```python
from build123d import *

# Parameters (mm, degrees)
SKETCH1_W            = 31.75
SKETCH1_H            = 50.8
BOSS_EXTRUDE1_DEPTH  = 3.175
CUT_EXTRUDE1_REACH   = 32.121
SKETCH2_R            = 12.7
M4_CLEARANCE_HOLE1_D = 4.4958


with BuildPart() as part:
    # Sketch1 → Boss-Extrude1 (new body)
    with BuildSketch(Plane(origin=(0, 0, 0), x_dir=(1, 0, 0), z_dir=(0, 1, 0))):
        Rectangle(SKETCH1_W, SKETCH1_H)
    extrude(amount=BOSS_EXTRUDE1_DEPTH)

    # Sketch2 → Cut-Extrude1 (cut, up to next)
    with BuildSketch(Plane(origin=(0, 3.175, 0), x_dir=(1, 0, 0), z_dir=(0, 1, 0)), mode=Mode.PRIVATE) as cut_extrude1_sk1:
        with Locations(Location((0, 0, 0), (0, 0, 270))):
            Circle(SKETCH2_R)
    cut_extrude1_tool1 = extrude(cut_extrude1_sk1.sketch, amount=-CUT_EXTRUDE1_REACH, mode=Mode.PRIVATE) & part.part
    add(cut_extrude1_tool1.solids().sort_by_distance((0, 3.175, 0))[0], mode=Mode.SUBTRACT)

    # M4 Clearance Hole1 (through all)
    with Locations(Plane(origin=(0, 3.175, 0), x_dir=(1, 0, 0), z_dir=(0, 1, 0))):
        with Locations((12.374792935, -12.374792935), (-12.374792935, -12.374792935), (-12.374792935, 12.374792935), (12.374792935, 12.374792935)):
            Hole(M4_CLEARANCE_HOLE1_D / 2)


solid = part.part
```
Geometry check sheet. Reference: the model listing, model coordinates, mm. Coordinates: 2 decimals unless noted, no trailing zeros. Order: outer loops, then holes, each group sorted by start corner. A loop starts at its lowest first (then second) coordinate and runs counter-clockwise, first axis right, second up.
Q1. Sectioned sample at B-B on z = 0. Record the cut outline in (x, y) (3 decimals).
Reply:
outline: (-15.875, 0) - (-12.7, 0) - (-12.7, 3.175) - (-15.875, 3.175) - close; (12.7, 0) - (15.875, 0) - (15.875, 3.175) - (12.7, 3.175) - close
Q2. Sectioned sample at D-D on x = 13.5. Record the cut outline in (y, z) (3 decimals), and give its area (3 significant figures).
Reply:
outline: (0, -25.4) - (3.175, -25.4) - (3.175, -14.321) - (0, -14.321) - close; (0, -10.429) - (3.175, -10.429) - (3.175, 10.429) - (0, 10.429) - close; (0, 14.321) - (3.175, 14.321) - (3.175, 25.4) - (0, 25.4) - close
area: 137 mm2
Q3. Depth check by flat-ended pin: pin 1 Ø3.5 at (x, z) = (12.37, -12.37) entering from -Y. Enter the tip coordinate at first touch or a pass-through.
Reply:
pin 1: passes through
Q4. Thickness scan on probe 1 along Z at (x, y) = (10.5, 1.45); probe 2 along X at (y, z) = (1.65, 14) (3 decimals); probe 3 along X at (y, z) = (2.35, 0) (3 decimals). Record the ranges inside material, lowest first.
Reply:
probe 1: z = -25.4 to -13.62, -11.13 to -7.14, 7.14 to 11.13, 13.62 to 25.4
probe 2: x = -15.875 to -13.928, -10.822 to 10.822, 13.928 to 15.875
probe 3: x = -15.875 to -12.7, 12.7 to 15.875
Q5. Sectioned sample at C-C on y = 1.9. Record the cut outline in (x, z) (3 decimals), and give its area (3 significant figures).
Reply:
outline: (-15.875, -25.4) - (15.875, -25.4) - (15.875, 25.4) - (-15.875, 25.4) - close; hole circle Ø4.496 at (-12.375, -12.375); hole circle Ø4.496 at (-12.375, 12.375); hole circle Ø25.4 at (0, 0); hole circle Ø4.496 at (12.375, -12.375); hole circle Ø4.496 at (12.375, 12.375)
area: 1,040 mm2
Q6. Draft check along Z on faces 1 (the face through (14.62, 1.57, -12.47)), 2 (the face through (0, 2, 25.4)), 3 (the face through (-7, 0, 11)), 4 (the face through (0, 2, -25.4)). Enter one of: released by +Z, released by -Z, zero draft, split by the parting line, or undercut.
Reply:
face 1: undercut
face 2: released by +Z
face 3: zero draft
face 4: released by -Z
Q7. Sectioned sample at A-A on x = 0. Record the cut outline in (y, z) (3 decimals), and give its area (3 significant figures).
Reply:
outline: (0, -25.4) - (3.175, -25.4) - (3.175, -12.7) - (0, -12.7) - close; (0, 12.7) - (3.175, 12.7) - (3.175, 25.4) - (0, 25.4) - close
area: 80.6 mm2
